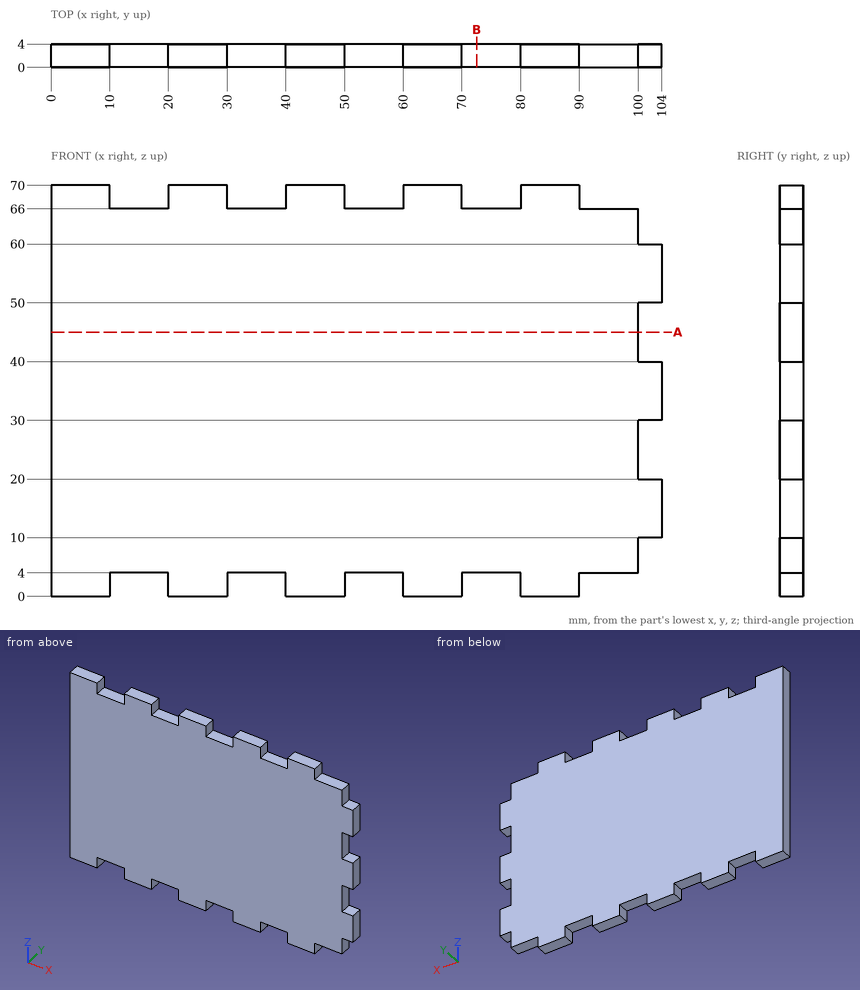
The figure shows three views and two pictorial views of one solid part (mm, origin at its lowest corner). Answer the questions. Coordinates: 2 decimals unless noted, no trailing zeros. Order: outer loops, then holes, each group sorted by start corner. A loop starts at its lowest first (then second) coordinate and runs counter-clockwise, first axis right, second up. Notation, with made-up numbers: (-25.5, -2) - (-21.5, -2) arc R6 cw to (-21.5, 9) - close; hole circle Ø8 at (-22.75, 53.25). An arc over 180 degrees is marked (long way). Answer as a JSON object with one key per item and string values.
1. Consider line 1 (Z direction, x = 38, y = 1.75); line 2 (X direction, y = 1.05, z = 62.5). Determine where each line is inside the solid, lowest interval first.
Output values:
{"line 1": "z = 4 to 66", "line 2": "x = 0 to 100"}
2. Find section B-B on x = 72.5. Determine the outline of the cut face in (y, z), plus the area to 3 significant figures.
Output values:
{"outline": "(0, 4) - (4, 4) - (4, 66) - (0, 66) - close", "area": "248 mm²"}
3. Each of these flat-tipped pins is pushed along its axis until it touches: P1, Ø1.2, axis at y = 2, z = 2, coming from the +X side; P2, Ø2, axis at y = 3, z = 6, coming from the +X side; P3, Ø1.2, axis at x = 75, y = 2.5, coming from the -Z side. Where does it stop, or does it pass through?
Output values:
{"P1": "stops at x = 90", "P2": "stops at x = 100", "P3": "stops at z = 4"}
4. Find section A-A on z = 45. Determine the outline of the cut face in (x, y).
Output values:
{"outline": "(0, 0) - (100, 0) - (100, 4) - (0, 4) - close"}
